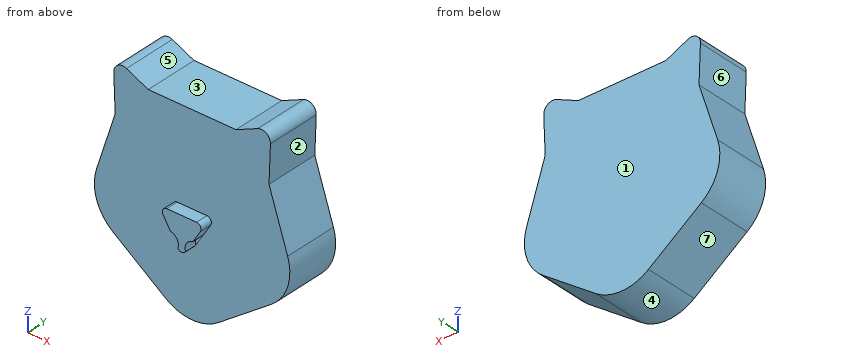
```python
from build123d import *

# Parameters (mm, degrees)
F1_DEPTH  = 6
F3_DEPTH  = 6
F5_R      = 2
F6_R      = 10
F9_DEPTH  = 2.7195
F10_R     = 1
F18_DEPTH = 2.7


# Not quite as in the source:
# - the program builds the solid bodies; features that only make, move or delete a surface that nothing else refers to are left out


with BuildPart() as f1:
    # F0 (on Front) → F1 (new body, symmetric)
    with BuildSketch(Plane.XZ):
        Polygon((-23.5114100917, -7.639320225), (0, -24.72135955), (23.5114100917, -7.639320225), (14.5308505601, 20), (-14.5308505601, 20), align=None)
    extrude(amount=F1_DEPTH, both=True)

    # F2 (on Front) → F3 (join, symmetric)
    with BuildSketch(Plane.XZ):
        Polygon((-17.5627600402, 23.5819537193), (-17.116108973, 12.0433927434), (-9.7525370519, 20), align=None)
        Polygon((17.5627600402, 23.5819537193), (9.7525370519, 20), (17.116108973, 12.0433927434), align=None)
    extrude(amount=F3_DEPTH, both=True)

    # F5
    f5_edges = [f1.edges().sort_by_distance(p)[0] for p in [
        (-17.56276, 0, 23.581954),
        (17.56276, 0, 23.581954),
    ]]
    fillet(f5_edges, radius=F5_R)

    # F6
    f6_edges = [f1.edges().sort_by_distance(p)[0] for p in [
        (-23.51141, 0, -7.63932),
        (23.51141, 0, -7.63932),
        (0, 0, -24.72136),
    ]]
    fillet(f6_edges, radius=F6_R)

    # F8 (on face) → F9 (join)
    with BuildSketch(Plane.XZ.offset(6)):
        Polygon((5.0926953554, 0), (-5.0926953554, 0), (0, -8.3154477179), align=None)
    extrude(amount=F9_DEPTH)

    # F10
    f10_edges = [f1.edges().sort_by_distance(p)[0] for p in [
        (0, -7.35975, -8.315448),
        (-5.092695, -7.35975, 0),
        (5.092695, -7.35975, 0),
    ]]
    fillet(f10_edges, radius=F10_R)

    # F17 (on face) → F18 (cut)
    with BuildSketch(Plane.XZ.offset(8.7195)):
        with BuildLine():
            Line((0.8527780007, -6.9230159338), (2.5065876623, -4.2226447518))
            ThreePointArc((2.5065876623, -4.2226447518), (1.0499427142, -5.1871536265), (0.8527780007, -6.9230159338))
        make_face()
        with BuildLine():
            Line((-2.5065876623, -4.2226447518), (-0.8527780007, -6.9230159338))
            ThreePointArc((-0.8527780007, -6.9230159338), (-1.0499427142, -5.1871536265), (-2.5065876623, -4.2226447518))
        make_face()
    extrude(amount=-F18_DEPTH, mode=Mode.SUBTRACT)


solid = f1.part
```
Check sheet for the modelled part. Datum: model origin and axes. Units: mm. Face numbers are marked on the shaded views. A direction names the side the tool comes from. Round coordinates to 2 decimals unless told otherwise and drop trailing zeros. Loops run counter-clockwise (first coordinate to the right, second up) from the corner with the lowest first, then second, coordinate; pieces in that order, holes last. Notation, with made-up numbers: (-39, 37.5) - (-17, 37.5) arc R10 cw to (-17, 50.5) - close; hole circle Ø7 at (42.25, 0.5). An arc over 180 degrees is marked (long way). Write item = value, one per line. Start each with the question number.
Q1. Access from +Z, -Z, +X, -X, +Y, -Y to the whole of each face (thin tool, end or side, straight path). Record for the marked faces 5, 6 and 7.
Q2. Section check B-B (z = -18.5). Record the boundary of the cut face in (x, y).
Q3. Section check A-A (y = -2.25). Record the boundary of the cut face in (x, z).
Q4. Depth check by flat-ended pin: P1, Ø0.9, axis at x = 1.5, z = -6, coming from the -Y side; P2, Ø1, axis at y = 0, z = -1.5, coming from the +X side; P3, Ø1, axis at x = 14.5, y = 3, coming from the -Z side; P4, Ø1.9, axis at x = -1.5, z = -5, coming from the -Y side. Enter the tip coordinate at first touch or a pass-through.
Q5. Thickness scan on L1, parallel to X at y = 4.25, z = -3.5; L2, parallel to Y at x = 14, z = 1.5; L3, parallel to Z at x = 1, y = -0.25. Record the ranges inside material, lowest first.
Q6. Release check for a two-part mould opening along Z. For the marked faces 1, 2, 3 and 4 record: pulls with the +Z half, pulls with the -Z half, needs draft (parallel to the pull), parting line crosses it, or undercut.
Q7. Section check C-C (x = -13.5). Record the boundary of the cut face in (y, z), plus the area to 3 significant figures.
Derived:
q1.face_5 = +Z, +Y, -Y
q1.face_6 = -X, +Y, -Y
q1.face_7 = -Z, -X, +Y, -Y
q2.outline = (-8.56, -6) - (8.56, -6) - (8.56, 6) - (-8.56, 6) - close
q3.outline = (-21.27, -0.73) arc R10 ccw to (-17.63, -11.91) - (-5.88, -20.45) arc R10 ccw to (5.88, -20.45) - (17.63, -11.91) arc R10 ccw to (21.27, -0.73) - (17.12, 12.04) - (17.44, 20.33) arc R2 ccw to (14.6, 22.23) - (9.75, 20) - (-9.75, 20) - (-14.6, 22.23) arc R2 ccw to (-17.44, 20.33) - (-17.12, 12.04) - close
q4.P1 = -6.02
q4.P2 = 21.59
q4.P3 = -14.55
q4.P4 = -8.72
q5.L1 = -21.75 to 21.75
q5.L2 = -6 to 6
q5.L3 = -22.31 to 20
q6.face_1 = needs draft
q6.face_2 = undercut
q6.face_3 = pulls with the +Z half
q6.face_4 = pulls with the -Z half
q7.outline = (-6, -14.91) - (6, -14.91) - (6, 21.72) - (-6, 21.72) - close
q7.area = 440 mm^2
